```python
from build123d import *

# Parameters (mm, degrees)
SKETCH1_W               = 86
SKETCH1_H               = 86
SKETCH1_W_2             = 80
SKETCH1_H_2             = 80
EXTRUDE_THIN1_DEPTH     = 6
CUT_EXTRUDE1_DEPTH      = 94.669632219
CUT_EXTRUDE1_DEPTH_BACK = 94.669632219
SKETCH2_R               = 1.5


with BuildPart() as part:
    # Sketch1 → Extrude-Thin1 (new body)
    with BuildSketch(Plane(origin=(0, 0, 0), x_dir=(1, 0, 0), z_dir=(0, 1, 0))):
        with Locations((-0.220557938, 0)):
            Rectangle(SKETCH1_W, SKETCH1_H)
        with Locations((-0.220557938, 0)):
            Rectangle(SKETCH1_W_2, SKETCH1_H_2, mode=Mode.SUBTRACT)
    extrude(amount=EXTRUDE_THIN1_DEPTH)

    # Sketch2 → Cut-Extrude1 (cut, two sides: drawn at the far end of the back side and taken through both)
    with BuildSketch(Plane.ZY.offset(-39.779442062).offset(-CUT_EXTRUDE1_DEPTH_BACK)):
        with Locations((0, 3)):
            Circle(SKETCH2_R)
    extrude(amount=CUT_EXTRUDE1_DEPTH + CUT_EXTRUDE1_DEPTH_BACK, mode=Mode.SUBTRACT)


solid = part.part
```
Input: part model. Units: mm. Frame: model coordinates. A direction names the side the tool comes from. Round coordinates to 2 decimals unless told otherwise and drop trailing zeros. Loops run counter-clockwise (first coordinate to the right, second up) from the corner with the lowest first, then second, coordinate; pieces in that order, holes last. Notation, with made-up numbers: M 65.5,-0.75 L 112.5,-0.75 A28 cw 112.5,21.25 Z; hole C 9,-24.75 d1. An arc over 180 degrees is marked long. Answer in a Markdown table with one row per item. Add a question column.
1. Section A-A (x = -2.5). Output: boundary loops of the cut face in (y, z), and give its area (3 significant figures).
2. Section B-B (z = 0). Output: boundary loops of the cut face in (x, y), and give its area (3 significant figures).
3. Section C-C (y = 3). Output: boundary loops of the cut face in (x, z).
4. Set-up query: faces 1 (the face through (-4, 0, 41)), 2 (the face through (-40.221, 1, 1)). Return all of +Z, -Z, +X, -X, +Y, -Y with unobstructed straight access to the full face (end or side cutting, diameter ignored); none if empty.
5. Ray query, probe 1 along X at (y, z) = (2.65, 4.5); probe 2 along Y at (x, z) = (-42, 0); probe 3 along Z at (x, y) = (-41.9, 3). Return the intervals inside material, ascending.
6. Mould query, pull axis X, two halves, no side actions, for faces 3 (the face through (-1, 3, 40)), 4 (the face through (-41.7, 1.536, -0.325)), 5 (the face through (-43.221, 1, 1)). Classes: released by +X, released by -X, zero draft, split by the parting line, or undercut.
7. Section D-D (z = 31). Output: boundary loops of the cut face in (x, y), and give its area (3 significant figures).
Values follow:
| question | item | result |
|---|---|---|
| 1 | outline | M 0,-43 L 6,-43 L 6,-40 L 0,-40 Z; M 0,40 L 6,40 L 6,43 L 0,43 Z |
| 1 | area | 36.0 mm^2 |
| 2 | outline | M -43.22,0 L -40.22,0 L -40.22,1.5 L -43.22,1.5 Z; M -43.22,4.5 L -40.22,4.5 L -40.22,6 L -43.22,6 Z; M 39.78,0 L 42.78,0 L 42.78,1.5 L 39.78,1.5 Z; M 39.78,4.5 L 42.78,4.5 L 42.78,6 L 39.78,6 Z |
| 2 | area | 18.0 mm^2 |
| 3 | outline | M -43.22,-43 L 42.78,-43 L 42.78,-1.5 L 39.78,-1.5 L 39.78,-40 L -40.22,-40 L -40.22,-1.5 L -43.22,-1.5 Z; M -43.22,1.5 L -40.22,1.5 L -40.22,40 L 39.78,40 L 39.78,1.5 L 42.78,1.5 L 42.78,43 L -43.22,43 Z |
| 4 | face 1 | +Z, -Z, +X, -X, -Y |
| 4 | face 2 | +Y, -Y |
| 5 | probe 1 | -43.22 to -40.22, 39.78 to 42.78 |
| 5 | probe 2 | 0 to 1.5, 4.5 to 6 |
| 5 | probe 3 | -43 to -1.5, 1.5 to 43 |
| 6 | face 3 | undercut |
| 6 | face 4 | zero draft |
| 6 | face 5 | released by -X |
| 7 | outline | M -43.22,0 L -40.22,0 L -40.22,6 L -43.22,6 Z; M 39.78,0 L 42.78,0 L 42.78,6 L 39.78,6 Z |
| 7 | area | 36.0 mm^2 |
